```python
from build123d import *

# Parameters (mm, degrees)
BOSS_EXTRUDE1_DEPTH = 6.5
SKETCH2_R           = 3.1
CUT_EXTRUDE1_DEPTH  = 24.228931445
SKETCH3_R           = 1.75
BOSS_EXTRUDE2_DEPTH = 2
CUT_EXTRUDE2_DEPTH  = 4.5
FILLET1_R           = 10
FILLET2_R           = 2


with BuildPart() as part:
    # Sketch1 → Boss-Extrude1 (new body)
    with BuildSketch(Plane(origin=(0, 0, 0), x_dir=(1, 0, 0), z_dir=(0, 1, 0))):
        with BuildLine():
            Line((-6.489945331, 18.917732676), (0, 5))
            Line((0, 5), (6.489945331, 18.917732676))
            ThreePointArc((6.489945331, 18.917732676), (9.254177969, 17.730205586), (11.809007007, 16.141479285))
            Line((11.809007007, 16.141479285), (6, 3.684023558))
            Line((6, 3.684023558), (6, -6))
            Line((6, -6), (-6, -6))
            Line((-6, -6), (-6, 3.684023558))
            Line((-6, 3.684023558), (-11.809007007, 16.141479285))
            ThreePointArc((-11.809007007, 16.141479285), (-9.254177969, 17.730205586), (-6.489945331, 18.917732676))
        make_face()
    extrude(amount=BOSS_EXTRUDE1_DEPTH)

    # Sketch2 → Cut-Extrude1 (cut, through all)
    with BuildSketch(Plane.XZ):
        with Locations(Location((0, 0, 0), (0, 0, 270))):
            Circle(SKETCH2_R)
    extrude(amount=-CUT_EXTRUDE1_DEPTH, mode=Mode.SUBTRACT)

    # Sketch3 → Boss-Extrude2 (add)
    # profile 1 of 2: a face of its own
    with BuildSketch(Plane(origin=(0, 6.5, 0), x_dir=(1, 0, 0), z_dir=(0, 1, 0))):
        with BuildLine():
            Line((12.285151677, 19.938771315), (11.809007007, 16.141479285))
            Line((11.809007007, 16.141479285), (8.152317162, 17.179463846))
            ThreePointArc((8.152317162, 17.179463846), (7.638707607, 22.42342918), (12.285151677, 19.938771315))
        make_face()
        with Locations(Location((9.297601758, 19.938771315, 0), (0, 0, 270))):
            Circle(SKETCH3_R, mode=Mode.SUBTRACT)
    # profile 2 of 2: a face of its own
    with BuildSketch(Plane(origin=(0, 6.5, 0), x_dir=(1, 0, 0), z_dir=(0, 1, 0))):
        with BuildLine():
            Line((-11.809007007, 16.141479285), (-8.152317162, 17.179463846))
            ThreePointArc((-8.152317162, 17.179463846), (-7.638707607, 22.42342918), (-12.285151677, 19.938771315))
            Line((-12.285151677, 19.938771315), (-11.809007007, 16.141479285))
        make_face()
        with Locations(Location((-9.297601758, 19.938771315, 0), (0, 0, 90))):
            Circle(SKETCH3_R, mode=Mode.SUBTRACT)
    extrude(amount=-BOSS_EXTRUDE2_DEPTH)

    # Sketch5 → Cut-Extrude2 (cut)
    with BuildSketch(Plane.XZ):
        with BuildLine():
            ThreePointArc((10.849326324, -16.801551069), (8.221259471, -16.608382857), (6.203329268, -18.303082545))
            Line((6.203329268, -18.303082545), (6.489945331, -18.917732676))
            ThreePointArc((6.489945331, -18.917732676), (8.733964823, -17.992161028), (10.849326324, -16.801551069))
        make_face()
        with BuildLine():
            Line((6.489945331, -18.917732676), (6.203329268, -18.303082545))
            ThreePointArc((6.203329268, -18.303082545), (8.454973049, -23.335825459), (12.797601758, -19.938771315))
            ThreePointArc((12.797601758, -19.938771315), (12.270902616, -18.092293043), (10.849326324, -16.801551069))
            ThreePointArc((10.849326324, -16.801551069), (8.733964823, -17.992161028), (6.489945331, -18.917732676))
        make_face()
        with BuildLine():
            ThreePointArc((-10.849326324, -16.801551069), (-11.144080031, -22.912072172), (-5.797601758, -19.938771315))
            ThreePointArc((-5.797601758, -19.938771315), (-5.900547614, -19.096142606), (-6.203329268, -18.303082545))
            Line((-6.203329268, -18.303082545), (-6.489945331, -18.917732676))
            ThreePointArc((-6.489945331, -18.917732676), (-8.733964823, -17.992161028), (-10.849326324, -16.801551069))
        make_face()
        with BuildLine():
            Line((-6.489945331, -18.917732676), (-6.203329268, -18.303082545))
            ThreePointArc((-6.203329268, -18.303082545), (-8.221259471, -16.608382857), (-10.849326324, -16.801551069))
            ThreePointArc((-10.849326324, -16.801551069), (-8.733964823, -17.992161028), (-6.489945331, -18.917732676))
        make_face()
    extrude(amount=-CUT_EXTRUDE2_DEPTH, mode=Mode.SUBTRACT)

    # Fillet1
    # the kernel refuses this fillet: 10 mm, written as the material it takes off along each edge
    with BuildSketch(Plane(origin=(6, -24.987516744, 6), x_dir=(-1, 0, 0), z_dir=(0, 1, 0))) as fillet1_piece_1:
        with BuildLine():
            CenterArc((9.995006698, -10), FILLET1_R, 90, 88.189286954)
            Line((0, -9.684023558), (-0.199900134, -9.677704029))
            ThreePointArc((-0.199900134, -9.677704029), (-0.2, -4.842011779), (-0.2, 0))
            Line((-0.2, 0), (0, 0.2))
            Line((0, 0.2), (9.995006698, 0.2))
            Line((9.995006698, 0.2), (9.995006698, 0))
        make_face()
    extrude(amount=56.475033489, mode=Mode.SUBTRACT)
    with BuildSketch(Plane(origin=(-6, -24.987516744, 6), x_dir=(0, 0, -1), z_dir=(0, 1, 0))) as fillet1_piece_2:
        with BuildLine():
            CenterArc((10, -9.995006698), FILLET1_R, 91.810713046, 88.189286954)
            Line((0, -9.995006698), (-0.2, -9.995006698))
            Line((-0.2, -9.995006698), (-0.2, 0))
            Line((-0.2, 0), (0, 0.2))
            ThreePointArc((0, 0.2), (4.842011779, 0.2), (9.677704029, 0.199900134))
            Line((9.677704029, 0.199900134), (9.684023558, 0))
        make_face()
    extrude(amount=56.475033489, mode=Mode.SUBTRACT)

    # Fillet2
    fillet2_edges = [part.edges().sort_by_distance(p)[0] for p in [
        (0, 3.25, -5),
    ]]
    fillet(fillet2_edges, radius=FILLET2_R)


solid = part.part
```
Geometry check sheet. Reference: the model listing, model coordinates, mm. A direction names the side the tool comes from. Coordinates: 2 decimals unless noted, no trailing zeros. Order: outer loops, then holes, each group sorted by start corner. A loop starts at its lowest first (then second) coordinate and runs counter-clockwise, first axis right, second up. Notation, with made-up numbers: M 75,72.5 L 134,72.5 A26 ccw 134,95.5 Z; hole C 7.5,31.5 d10. An arc over 180 degrees is marked long. Answer as a JSON object with one key per item and string values.
Q1. Cross-section at D-D on x = -8. Record the cut outline in (y, z), and give its area (3 significant figures).
Results are:
{"outline": "M 0,-16.69 L 4.5,-16.69 L 4.5,-18.76 L 6.5,-18.76 L 6.5,-7.97 L 0,-7.97 Z; M 4.5,-22.63 L 6.5,-22.63 L 6.5,-21.11 L 4.5,-21.11 Z", "area": "63.8 mm²"}
Q2. Depth check by flat-ended pin: pin 1 Ø3 at (x, z) = (-9.3, -19.94) entering from -Y; pin 2 Ø1 at (y, z) = (5, 1) entering from -X; pin 3 Ø5 at (x, z) = (10, -21) entering from -Y. Enter the tip coordinate at first touch or a pass-through.
Results are:
{"pin 1": "passes through", "pin 2": "stops at x = -4.94", "pin 3": "stops at y = 4.5"}
Q3. Release check for a two-part mould opening along Z. For faces 1 (the cylindrical face through (-11.3, 2.2, -16.5)), 2 (the cylindrical face through (-4.327, 3.204, 1.545)), 3 (the cylindrical face through (-11.033, 5.514, -19.711)) record: released by +Z, released by -Z, zero draft, split by the parting line, or undercut.
Results are:
{"face 1": "released by -Z", "face 2": "released by +Z", "face 3": "undercut"}
Q4. Cross-section at B-B on x = -2.25. Record the cut outline in (y, z), and give its area (3 significant figures).
Results are:
{"outline": "M 0,-9.83 L 6.5,-9.83 L 6.5,-2.13 L 0,-2.13 Z; M 0,2.13 L 6.5,2.13 L 6.5,3.81 L 0,3.81 Z", "area": "60.9 mm²"}
Q5. Cross-section at C-C on y = 2.5. Record the cut outline in (x, z) (3 decimals), and give its area (3 significant figures).
Results are:
{"outline": "M -11.809,-16.141 A20 ccw -10.849,-16.802 A3.5 cw -6.203,-18.303 L -1.813,-8.887 A2 cw 1.813,-8.887 L 6.203,-18.303 A3.5 cw 10.849,-16.802 A20 ccw 11.809,-16.141 L 6,-3.684 A10 ccw 0,5.167 A10 ccw -6,-3.684 Z; hole C 0,0 d6.2", "area": "223 mm²"}
Q6. Tool access check on faces 4 (the flat face through (0, 0, -7)), 5 (the cylindrical face through (8.257, 2.218, -16.597)). Record the directions out of +Z, -Z, +X, -X, +Y, -Y that give a thin tool (end or side, any length) a straight path to the whole face; none if there is none.
Results are:
{"face 4": "+Z, -Z, +X, -X, -Y", "face 5": "-Z, -Y"}
Q7. Scan lines: line 1 (Z direction, x = 2.25, y = 4); line 2 (X direction, y = 3.75, z = 2.75); line 3 (X direction, y = 6, z = -14.25). Record each from-to range of solid material in increasing order.
Results are:
{"line 1": "z = -9.83 to -2.13, 2.13 to 3.81", "line 2": "x = -3.38 to -1.43, 1.43 to 3.38", "line 3": "x = -10.93 to -4.31, 4.31 to 10.93"}
Q8. Cross-section at A-A on z = -14.75. Record the cut outline in (x, y).
Results are:
{"outline": "M -11.16,0 L -4.55,0 L -4.55,6.5 L -11.16,6.5 Z; M 4.55,0 L 11.16,0 L 11.16,6.5 L 4.55,6.5 Z"}
